Source: three-view drawing plus pictorial views. Frame: mm from the lowest corner of the part. A direction names the side the tool comes from. Coordinates: 2 decimals unless noted, no trailing zeros. Write each loop counter-clockwise with the first axis right and the second up, starting at its lowest first coordinate (ties: lowest second). Pieces come first, ordered by that corner, then holes. Notation, with made-up numbers: (-15, -20) -> (19, -20) arc R29 ccw to (19, 17) -> close; hole circle Ø5 at (5.5, -9). An arc over 180 degrees is marked (long way). One line per item, written item: value.
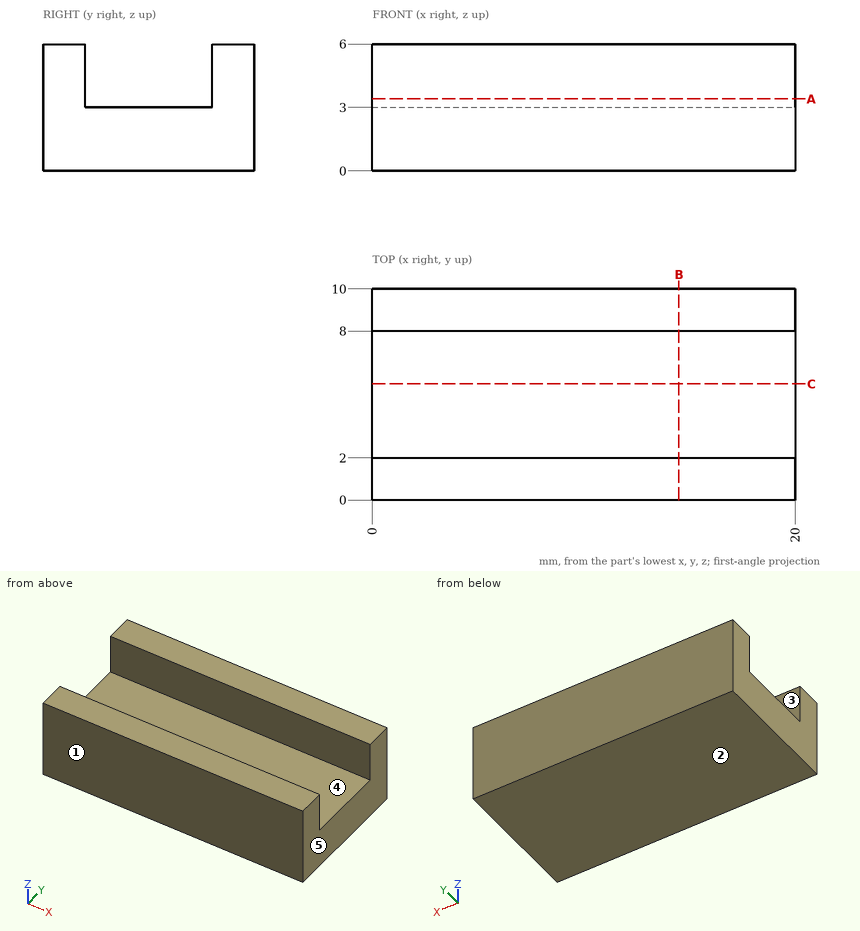
(1) Pull-direction query (Y, two-part tool) for the marked faces 1, 2 and 3; classes: released by +Y, released by -Y, zero draft, split by the parting line, or undercut.
Responses:
face 1: released by -Y
face 2: zero draft
face 3: undercut
(2) Section B-B (x = 14.5). Return the cut outline in (y, z), then the cut area to 3 significant figures.
Responses:
outline: (0, 0) -> (10, 0) -> (10, 6) -> (8, 6) -> (8, 3) -> (2, 3) -> (2, 6) -> (0, 6) -> close
area: 42.0 mm2
(3) Line query: line 1 (Y direction, x = 6.75, z = 3.05); line 2 (Z direction, x = 18.5, y = 7.25). Output: solid intervals per line, ascending. Write a range as [from, to].
Responses:
line 1: y = [0, 2], [8, 10]
line 2: z = [0, 3]
(4) Reachability of the marked faces 4 and 5 from +Z, -Z, +X, -X, +Y, -Y: full face, straight path, thin tool, end or side. Return the list, or none.
Responses:
face 4: +Z, +X, -X
face 5: +Z, -Z, +X, +Y, -Y
(5) First-contact query: pin 1 (1.8 mm diameter, centred on x = 9.5, y = 6.5, fed in from +Z). Flat tip, straight axial feed; report the tip coordinate or a pass-through.
Responses:
pin 1: stops at z = 3
(6) Section A-A (z = 3.4). Return the cut outline in (x, y), then the cut area to 3 significant figures.
Responses:
outline: (0, 0) -> (20, 0) -> (20, 2) -> (0, 2) -> close; (0, 8) -> (20, 8) -> (20, 10) -> (0, 10) -> close
area: 80.0 mm2
(7) Section C-C (y = 5.5). Return the cut outline in (x, z).
Responses:
outline: (0, 0) -> (20, 0) -> (20, 3) -> (0, 3) -> close
